```python
from build123d import *

# Parameters (mm, degrees)
SKETCH1_R           = 21.082
SKETCH1_R_2         = 17.526
BOSS_EXTRUDE1_DEPTH = 965.2
CUT_EXTRUDE1_DEPTH  = 22.082
CUT_EXTRUDE2_DEPTH  = 22.0820001


with BuildPart() as part:
    # Sketch1 → Boss-Extrude1 (new body)
    with BuildSketch(Plane(origin=(0, 0, 0), x_dir=(0, 0, -1), z_dir=(1, 0, 0))):
        Circle(SKETCH1_R)
        Circle(SKETCH1_R_2, mode=Mode.SUBTRACT)
    extrude(amount=BOSS_EXTRUDE1_DEPTH)

    # Sketch2 → Cut-Extrude1 (cut, through all)
    with BuildSketch(Plane.XY):
        with BuildLine():
            Line((7.9375, 3.175), (20.6375, 3.175))
            ThreePointArc((20.6375, 3.175), (23.8125, 0), (20.6375, -3.175))
            Line((20.6375, -3.175), (7.9375, -3.175))
            ThreePointArc((7.9375, -3.175), (4.7625, 0), (7.9375, 3.175))
        make_face()
        with BuildLine():
            Line((46.0375, 3.175), (58.7375, 3.175))
            ThreePointArc((58.7375, 3.175), (61.9125, 0), (58.7375, -3.175))
            Line((58.7375, -3.175), (46.0375, -3.175))
            ThreePointArc((46.0375, -3.175), (42.8625, 0), (46.0375, 3.175))
        make_face()
    extrude(amount=-CUT_EXTRUDE1_DEPTH, mode=Mode.SUBTRACT)

    # Sketch3 → Cut-Extrude2 (cut, through all)
    with BuildSketch(Plane.XY):
        with BuildLine():
            Line((781.05, 3.175), (933.45, 3.175))
            ThreePointArc((933.45, 3.175), (935.69506403, 2.24506403), (936.625, 0))
            Line((936.625, 0), (936.625, -6.35))
            ThreePointArc((936.625, -6.35), (933.45, -9.525), (930.275, -6.35))
            Line((930.275, -6.35), (930.275, -3.175))
            Line((930.275, -3.175), (781.05, -3.175))
            ThreePointArc((781.05, -3.175), (777.875, 0), (781.05, 3.175))
        make_face()
    extrude(amount=CUT_EXTRUDE2_DEPTH, mode=Mode.SUBTRACT)


solid = part.part
```
Input: part model. Units: mm. Frame: model coordinates. Round coordinates to 2 decimals unless told otherwise and drop trailing zeros. Write each loop counter-clockwise with the first axis right and the second up, starting at its lowest first coordinate (ties: lowest second). Pieces come first, ordered by that corner, then holes. Notation, with made-up numbers: (32, 51) -> (40, 51) arc R24 ccw to (40, 66) -> close; hole circle Ø2 at (-27, 88). An arc over 180 degrees is marked (long way). Answer as CSV lines item,"result".
1. Section B-B (y = 10.5). Return the cut outline in (x, z), plus the area to 3 significant figures.
Geometry says:
outline,"(0, -18.28) -> (965.2, -18.28) -> (965.2, -14.03) -> (0, -14.03) -> close; (0, 14.03) -> (965.2, 14.03) -> (965.2, 18.28) -> (0, 18.28) -> close"
area,"8,200 mm^2"
2. Mould query, pull axis Z, two halves, no side actions, for faces 1 (the flat face through (0, 16, 8)), 2 (the cylindrical face through (475.84, 6.33, -20.11)), 3 (the cylindrical face through (475.84, 5.26, -16.72)). Classes: +Z half, -Z half, draft (parallel to the pull), parting line (faces both ways), or undercut.
Geometry says:
face 1,"draft"
face 2,"parting line"
face 3,"undercut"
3. Section C-C (x = 582.5). Return the cut outline in (y, z), plus the area to 3 significant figures.
Geometry says:
outline,"circle Ø42.16 at (0, 0); hole circle Ø35.05 at (0, 0)"
area,"431 mm^2"
4. Ray query, L1, parallel to Z at x = 342, y = 0; L2, parallel to Y at x = 778, z = 2. Return the intervals inside material, ascending. Write a range as [from, to].
Geometry says:
L1,"z = [-21.08, -17.53], [17.53, 21.08]"
L2,"y = [-20.99, -17.41], [17.41, 20.99]"
5. Contact query for flat-ended pins moving along their axis: P1, Ø3, axis at x = 858.5, z = 18.5, coming from the +Y side; P2, Ø8, axis at x = 671.5, z = -12.5, coming from the -Y side; P3, Ø4, axis at x = 835, z = 19.5, coming from the -Y side. Output: stop coordinate, or through.
Geometry says:
P1,"stops at y = 12.47"
P2,"stops at y = -19.29"
P3,"stops at y = -11.76"
6. Section A-A (z = 4). Return the cut outline in (x, y).
Geometry says:
outline,"(0, -20.7) -> (965.2, -20.7) -> (965.2, -17.06) -> (0, -17.06) -> close; (0, 17.06) -> (965.2, 17.06) -> (965.2, 20.7) -> (0, 20.7) -> close"
